Autodesk Inventor part; units mm, degrees
ref_plane "YZ Plane" through (0, 0, 0) normal (1, 0, 0) x (0, 1, 0)
ref_plane "XZ Plane" through (0, 0, 0) normal (0, 1, 0) x (-1, 0, 0)
ref_plane "XY Plane" through (0, 0, 0) normal (0, 0, 1) x (1, 0, 0)
sketch "Boceto1" plane through (0, 0, 0) normal (0, 1, 0) x (-1, 0, 0)
  line L0 (27.5, -17.5) -> (-27.5, -17.5)
  line L1 (-27.5, -17.5) -> (-27.5, 17.5)
  line L2 (-27.5, 17.5) -> (27.5, 17.5)
  line L3 (27.5, 17.5) -> (27.5, -17.5)
  line L4 (27.5, -17.5) -> (-27.5, 17.5) construction
  line L5 (-27.5, -17.5) -> (27.5, 17.5) construction
  point P0 (0, 0)
  dimension "d0" = 55
  dimension "d1" = 35
extrude "Extrusión1" add sketch "Boceto1" along normal blind 15
sketch "Boceto2" plane through (0, 15, 0) normal (0, 1, 0) x (1, 0, 0)
  line L0 (25.5, -15.5) -> (-25.5, -15.5)
  line L1 (-25.5, -15.5) -> (-25.5, 15.5)
  line L2 (-25.5, 15.5) -> (25.5, 15.5)
  line L3 (25.5, 15.5) -> (25.5, -15.5)
  line L4 (25.5, -15.5) -> (-25.5, 15.5) construction
  line L5 (-25.5, -15.5) -> (25.5, 15.5) construction
  point P0 (0, 0)
  dimension "d4" = 51
  dimension "d5" = 31
extrude "Extrusión2" cut sketch "Boceto2" against normal blind 13
sketch "Boceto3" plane through (-27.5, 0, -17.5) normal (-1, 0, 0) x (0, 0, 1)
  point P0 (17.5, 0)
sketch "Boceto4" plane through (0, 15, 0) normal (0, 1, 0) x (1, 0, 0)
  line L0 (-27.5, 17.5) -> (-27.5, -17.5)
  line L1 (-27.5, -17.5) -> (-29.5, -17.5)
  line L2 (-29.5, -17.5) -> (-29.5, 17.5)
  line L3 (-29.5, 17.5) -> (-27.5, 17.5)
  line L4 (-27.5, 17.5) -> (-27.5, -17.5)
  point P0 (0, 0)
  dimension "d8" = 2
extrude "Extrusión3" add sketch "Boceto4" against normal blind 15
sketch "Boceto5" plane through (-29.5, 15, -17.5) normal (-1, 0, 0) x (0, 0, 1)
  line L0 (35, 0) -> (0, 0)
  line L1 (0, 0) -> (9, 0)
  line L2 (9, 0) -> (9, -6.5)
  line L3 (2, -13) -> (33, -13)
  circle A0 centre (9, -6.5) radius 5.5
  point P0 (17.5, -15)
  dimension "d11" = 9
  dimension "d12" = 6.5
  dimension "d13" = 11
extrude "Extrusión4" cut sketch "Boceto5" against normal blind 2
sketch "Boceto6" plane through (-27.5, 8.5, -8.5) normal (-1, 0, 0) x (0, 0, 1)
  circle A0 centre (0, 0) radius 4
  point P0 (8.5, -8.5)
  dimension "d16" = 8
extrude "Extrusión5" cut sketch "Boceto6" against normal blind 2
sketch "Boceto7" plane through (0, 2, 0) normal (0, 1, 0) x (1, 0, 0)
  line L0 (-27.5, 3) -> (-27.5, 14)
  line L1 (-27.5, 3) -> (-27.5, 8.5)
  line L2 (-25.5, -15.5) -> (-25.5, 15.5)
  line L3 (-25.5, 8.5) -> (-25.5, 1.5)
  line L4 (-25.5, 15.5) -> (25.5, 15.5)
  line L5 (7.5, 15.5) -> (7.5, 14.5)
  line L6 (7.5, 14.5) -> (6.5, 14.5)
  line L7 (6.5, 14.5) -> (6.5, 15.5)
  line L8 (6.5, 1.5) -> (6.5, 2.5547)
  line L9 (6.5, 2.5547) -> (7.5, 2.5547)
  line L10 (7.5, 2.5547) -> (7.5, 0.5)
  line L11 (7.5, 0.5) -> (-5.5, 0.5)
  line L12 (-5.5, 0.5) -> (-5.5, 1.5)
  line L13 (-5.5, 1.5) -> (6.5, 1.5)
  point P0 (0, 0)
  dimension "d19" = 7
  dimension "d27" = 32
extrude "Extrusión6" add sketch "Boceto7" along normal blind 13 contours L8 L9 L10 L11 L12 L13
sketch "Boceto8" plane through (0, 2, 0) normal (0, 1, 0) x (1, 0, 0)
  line L0 (6.5, 1.5) -> (6.5, 2.5547)
  line L1 (-25.5, 15.5) -> (25.5, 15.5)
  line L2 (6.5, 15.5) -> (6.5, 14.5)
  line L3 (6.5, 14.5) -> (7.5, 14.5)
  line L4 (7.5, 14.5) -> (7.5, 15.5)
  point P0 (0, 0)
extrude "Extrusión7" add sketch "Boceto8" along normal blind 13
sketch "Boceto9" plane through (0, 15, 0) normal (0, 1, 0) x (1, 0, 0)
  line L0 (-29.5, -17.5) -> (27.5, -17.5)
  line L1 (27.5, -17.5) -> (27.5, -21.5)
  line L2 (27.5, -21.5) -> (-29.5, -21.5)
  line L3 (-29.5, -21.5) -> (-29.5, -17.5)
  point P0 (0, 0)
  dimension "d34" = 4
extrude "Extrusión8" add sketch "Boceto9" against normal blind 15
sketch "Boceto10" plane through (0, 15, 0) normal (0, 1, 0) x (1, 0, 0)
  line L0 (25.5, -15.5) -> (-25.5, -15.5)
  line L1 (-25.5, -15.5) -> (25.5, -15.5)
  line L2 (25.5, -15.5) -> (25.5, -19.5)
  line L3 (25.5, -19.5) -> (-25.5, -19.5)
  line L4 (-25.5, -19.5) -> (-25.5, -15.5)
  point P0 (0, 0)
  dimension "d37" = 4
extrude "Extrusión9" cut sketch "Boceto10" against normal blind 13
sketch "Boceto11" plane through (-29.5, 0, -17.5) normal (-1, 0, 0) x (0, 0, 1)
  line L0 (39, 15) -> (37, 15)
  line L1 (39, 15) -> (0, 15)
  line L2 (37, 15) -> (27, 15)
  line L3 (0, 0) -> (39, 0)
  line L4 (2, 2) -> (37, 2)
  line L5 (27, 5.5) -> (27, 8.5)
  line L6 (27, 5.5) -> (31, 5.5)
  line L7 (31, 5.5) -> (31, 2.5)
  line L8 (31, 2.5) -> (23, 2.5)
  line L9 (23, 2.5) -> (23, 5.5)
  line L10 (23, 5.5) -> (27, 5.5)
  point P0 (17.5, 0)
  dimension "d41" = 10
  dimension "d45" = 3
  dimension "d46" = 4
extrude "Extrusión10" cut sketch "Boceto11" against normal blind 4
sketch "Boceto12" plane through (-25.5, 2, -15.5) normal (1, 0, 0) x (0, 0, -1)
  line L0 (-29, 3.5) -> (-29, 0.5)
  line L1 (-29, 3.5) -> (-25, 3.5)
  line L2 (-29, 3.5) -> (-21, 3.5)
  line L3 (-25, 6.5) -> (-21, 6.5)
  line L4 (-21, 0.5) -> (-21, 3.5)
  line L5 (-21, 6.5) -> (-21, 3.5)
  line L6 (-21, 3.5) -> (-29, 3.5)
  line L7 (-29, 6.5) -> (-29, 3.2703)
  line L8 (-29, 6.5) -> (-25, 6.5)
  point P0 (-15.5, -2)
sketch "Boceto13" plane through (-25.5, 2, -15.5) normal (1, 0, 0) x (0, 0, -1)
  line L0 (-25, 3.524) -> (-34.5, 3.524)
  line L1 (-35, 13) -> (-35, 0)
  line L2 (-34.5, 3.524) -> (-34.5, 6.524)
  line L3 (-35, 13) -> (0, 13)
  line L4 (-34.5, 6.524) -> (-15.5, 6.524)
  line L5 (-15.5, 6.524) -> (-15.5, 3.524)
  line L6 (-35, 0) -> (0, 0)
  line L7 (-15.5, 3.524) -> (-25, 3.524)
  point P0 (-15.5, -2)
  dimension "d52" = 9.5
  dimension "d54" = 3
  dimension "d55" = 19
  dimension "d56" = 3
extrude "Extrusión11" cut sketch "Boceto13" against normal blind 2
sketch "Boceto14" plane through (27.5, 0, -17.5) normal (1, 0, 0) x (0, 0, -1)
  line L0 (0, 15) -> (0, 0)
  line L1 (0, 0) -> (-19.5, 0)
  line L2 (-39, 0) -> (0, 0)
  line L3 (-19.5, 0) -> (-19.5, 7.5)
  line L4 (-36.5, 8.524) -> (-17.5, 8.524)
  line L5 (-19.5, 7.5) -> (-24.5, 7.5)
  line L6 (-39, 15) -> (-39, 0)
  line L7 (-24.5, 7.5) -> (-24.5, 6.5)
  line L8 (-24.5, 6.5) -> (-14.5, 6.5)
  line L9 (-14.5, 6.5) -> (-14.5, 8.5)
  line L10 (-37, 15) -> (-2, 15)
  line L11 (-24.5, 6.5) -> (-24.5, 8.5)
  line L12 (-24.5, 8.5) -> (-14.5, 8.5)
  point P0 (-17.5, 0)
  dimension "d59" = 19.5
  dimension "d60" = 7.5
  dimension "d61" = 5
  dimension "d62" = 1
  dimension "d63" = 10
  dimension "d64" = 2
  dimension "d65" = 2
extrude "Extrusión12" cut sketch "Boceto14" against normal blind 3
sketch "Boceto15" plane through (0, 15, 0) normal (0, 1, 0) x (1, 0, 0)
  line L0 (27.5, -21.5) -> (-29.5, -21.5)
  line L1 (27.5, 17.5) -> (-29.5, 17.5)
  line L2 (-29.5, -21.5) -> (27.5, -21.5)
  line L3 (27.5, -21.5) -> (27.5, 17.5)
  line L4 (27.5, 17.5) -> (-29.5, 17.5)
  line L5 (27.5, -21.5) -> (27.5, 17.5)
  line L6 (27.5, 17.5) -> (27.5, 16.5)
  line L7 (26.5, 16.5) -> (-28.5, 16.5)
  line L8 (-28.5, -20.5) -> (26.5, -20.5)
  line L9 (26.5, -20.5) -> (26.5, 16.5)
  line L10 (-28.5, 16.5) -> (-29.5, 16.5)
  line L11 (-29.5, 17.5) -> (-29.5, -21.5)
  line L12 (27.5, 17.5) -> (-29.5, 17.5)
  line L13 (-29.5, 16.5) -> (-29.5, 17.5)
  line L14 (-28.5, -20.5) -> (-29.5, -20.5)
  line L15 (-29.5, -21.5) -> (-29.5, -20.5)
  point P0 (0, 0)
  dimension "d69" = 1
  dimension "d70" = 55
  dimension "d71" = 37
sketch "Boceto16" plane through (0, 15, 0) normal (0, 1, 0) x (1, 0, 0)
  point P0 (0, 0)
extrude "Extrusión13" cut sketch "Boceto15" against normal blind 3 contours L0 L11 L14 L8 L9 L7 L10 L1 L3
sketch "Boceto17" plane through (-29.5, 15, 20.5) normal (0, 0, 1) x (1, 0, 0)
  line L0 (0, 0) -> (56, 0)
  line L1 (56, 0) -> (56, -3)
  line L2 (0, 0) -> (56, 0)
  line L3 (56, 0) -> (56, -1.5)
  line L4 (56, -1.5) -> (0, -1.5)
  line L5 (0, -1.5) -> (0, 0)
  point P0 (29.5, -15)
extrude "Extrusión14" add sketch "Boceto17" along normal blind 1
sketch "Boceto18" plane through (26.5, 15, -16.5) normal (0, 0, -1) x (-1, 0, 0)
  line L0 (0, 0) -> (56, 0)
  line L1 (0, -1.5) -> (56, -1.5)
  line L2 (0, 0) -> (56, 0)
  line L3 (56, 0) -> (56, -1.5)
  line L4 (56, -1.5) -> (0, -1.5)
  line L5 (0, -1.5) -> (0, 0)
  point P0 (26.5, -15)
extrude "Extrusión15" add sketch "Boceto18" along normal blind 1
sketch "Boceto19" plane through (-29.5, 0, -17.5) normal (-1, 0, 0) x (0, 0, 1)
  line L0 (23, 2.5) -> (23, 5.5)
  line L1 (23, 5.5) -> (31, 5.5)
  line L2 (31, 5.5) -> (31, 8.5)
  line L3 (31, 8.5) -> (23, 8.5)
  line L4 (23, 8.5) -> (23, 5.5)
  point P0 (17.5, 0)
  dimension "d78" = 8
  dimension "d79" = 3
extrude "Extrusión16" cut sketch "Boceto19" against normal blind 6
sketch "Boceto20" plane through (-29.5, 0, -17.5) normal (-1, 0, 0) x (0, 0, 1)
  line L0 (23, 8.5) -> (23, 5.524)
  line L1 (23, 8.5) -> (22.5, 8.5)
  line L2 (24.5, 8.5) -> (14.5, 8.5)
  line L3 (22.5, 8.5) -> (22.5, 2.5)
  line L4 (22.5, 2.5) -> (31.5, 2.5)
  line L5 (23, 2.5) -> (31, 2.5)
  line L6 (31.5, 2.5) -> (31.5, 8.5)
  line L7 (31.5, 8.5) -> (22.5, 8.5)
  point P0 (17.5, 0)
  dimension "d82" = 0.5
  dimension "d83" = 6
  dimension "d84" = 9
  dimension "d85" = 6
extrude "Extrusión17" cut sketch "Boceto20" against normal blind 6
sketch "Boceto21" plane through (-25.5, 2, -15.5) normal (1, 0, 0) x (0, 0, -1)
  line L0 (-34.5, 6.524) -> (-15.5, 6.524)
  line L1 (-34.5, 6.524) -> (-34.5, 7.524)
  line L2 (-34.5, 7.524) -> (-15.5, 7.524)
  line L3 (-15.5, 7.524) -> (-15.5, 6.524)
  line L4 (-15.5, 6.524) -> (-34.5, 6.524)
  point P0 (-15.5, -2)
  dimension "d88" = 1
extrude "Extrusión18" cut sketch "Boceto21" against normal blind 2
sketch "Boceto22" plane through (26.5, 12, 20.5) normal (1, 0, 0) x (0, 0, -1)
  line L0 (0, 0) -> (37, 0)
  line L1 (37, 0) -> (37, 3)
  line L2 (-1, 3) -> (38, 3)
  line L3 (37, 3) -> (38, 3)
  line L4 (37, 0) -> (38, 0)
  line L5 (38, 3) -> (38, 0)
  line L6 (38, 0) -> (37, 0)
  line L7 (0, 1.5) -> (0, 0)
  line L8 (-1, 0) -> (-1, -12)
  line L9 (0, 0) -> (-1, 0)
  line L10 (-1, 0) -> (-1, 3)
  line L11 (0, 3) -> (0, 0)
  point P0 (20.5, -12)
extrude "Extrusión19" cut sketch "Boceto22" against normal blind 100 contours L9 L10 L2 L11 L7 | L1 L2 L5 L4
sketch "Boceto23" plane through (26.5, 15, 20.5) normal (1, 0, 0) x (0, 0, -1)
  line L0 (37, 0) -> (37, -3)
  line L1 (37, 0) -> (38, 0)
  line L2 (38, 0) -> (38.5, 0)
  line L3 (38.5, 0) -> (38.5, 1)
  line L4 (38.5, 1) -> (37, 1)
  line L5 (37, 1) -> (36, 1)
  line L6 (36, 1) -> (36, 0)
  line L7 (37, 0) -> (36, 0)
  line L8 (0, 0) -> (37, 0)
  point P0 (20.5, -15)
  dimension "d93" = 1
  dimension "d94" = 0.5
  dimension "d95" = 1
extrude "Extrusión20" add sketch "Boceto23" against normal blind 56
sketch "Boceto24" plane through (26.5, 15, 20.5) normal (1, 0, 0) x (0, 0, -1)
  line L0 (36, 0) -> (0, 0)
  line L1 (0, 0) -> (-1.5, 0)
  line L2 (-1.5, 0) -> (-1.5, 1)
  line L3 (-1.5, 1) -> (0.5, 1)
  line L4 (0.5, 1) -> (1, 1)
  line L5 (1, 0) -> (36, 0)
  line L6 (1, 1) -> (1, 0)
  line L7 (1, 0) -> (0, 0)
  point P0 (20.5, -15)
  dimension "d98" = 1.5
  dimension "d99" = 1
  dimension "d100" = 2
  dimension "d101" = 0.5
extrude "Extrusión21" add sketch "Boceto24" against normal blind 56
sketch "Boceto25" plane through (26.5, 15, 19.5) normal (1, 0, 0) x (0, 0, -1)
  line L0 (-2.5, 1) -> (0, 1)
  line L1 (-1, 0) -> (-2.5, 0)
  line L2 (-2.5, 1) -> (-2, 1)
  line L3 (-2, 1) -> (-2, 0)
  line L4 (-2, 0) -> (-2.5, 0)
  line L5 (-2.5, 0) -> (-2.5, 1)
  line L6 (37.5, 1) -> (35, 1)
  line L7 (36, 0) -> (37.5, 0)
  line L8 (37.5, 1) -> (37, 1)
  line L9 (37, 1) -> (37, 0)
  line L10 (37, 0) -> (37.5, 0)
  line L11 (37.5, 0) -> (37.5, 1)
  point P0 (19.5, -15)
  point P1 (-2, 1)
  dimension "d104" = 0.5
  dimension "d105" = 0.5
extrude "Extrusión22" cut sketch "Boceto25" against normal blind 56
sketch "Boceto26" plane through (26.5, 15, 19.5) normal (1, 0, 0) x (0, 0, -1)
  point P0 (19.5, -15)
sketch "Boceto27" plane through (26.5, 15, 19.5) normal (1, 0, 0) x (0, 0, -1)
  line L0 (35, 0) -> (0, 0)
  line L1 (0, 1) -> (0, 0)
  line L2 (35, 0) -> (0, 0)
  line L3 (0, 0) -> (0, 1)
  line L4 (0, 1) -> (35, 1)
  line L5 (35, 1) -> (35, 0)
  point P0 (19.5, -15)
extrude "Extrusión23" add sketch "Boceto27" against normal blind 1
properties part number "CajaArduinoNano"
Geometry check sheet. Reference: the model listing, model coordinates, mm. A direction names the side the tool comes from. Coordinates: 2 decimals unless noted, no trailing zeros. Order: outer loops, then holes, each group sorted by start corner. A loop starts at its lowest first (then second) coordinate and runs counter-clockwise, first axis right, second up. Notation, with made-up numbers: (66.5, 28.25) - (95.5, 28.25) arc R25 ccw to (95.5, 43.25) - close; hole circle Ø4 at (20.25, -17.5). An arc over 180 degrees is marked (long way). Answer in a Markdown table with one row per item. Add a question column.
1) Gauge pin test, flat ends, axial feed: P1, Ø1.5, axis at x = -10, z = -1.5, coming from the +Y side; P2, Ø3, axis at x = -27, z = 9.5, coming from the +Y side; P3, Ø5, axis at y = 8.5, z = -8.5, coming from the -X side. Record the tip position at first contact, or that the pin passes through.
2) Cross-section at C-C, the plane z = 15.5. Record the cut outline in (x, y).
3) Cross-section at B-B, the plane x = 16. Record the cut outline in (y, z), then the cut area to 3 significant figures.
4) Material ranges on line 1 along X through (y, z) = (11.75, -15); line 2 along X through (y, z) = (12.5, 3); line 3 along X through (y, z) = (8, -13), recorded low to high. Write a range as [from, to].
5) Set-up check for faces 1 (the flat face through (25.5, 9, 2)), 2 (the flat face through (1, 15, -1)), 3 (the flat face through (-27.5, 4, -8)): record each of +Z, -Z, +X, -X, +Y, -Y from which the full face is reachable in a straight line by a thin tool's end or side.
6) Release check for a two-part mould opening along Z. For faces 4 (the flat face through (-26, 9.524, 10)), 5 (the flat face through (-1, 0, 2)), 6 (the flat face through (-1, 14, 20.5)) record: +Z half, -Z half, draft (parallel to the pull), parting line (faces both ways), or undercut.
7) Cross-section at D-D, the plane z = -8.5. Record the cut outline in (x, y), then the cut area to 3 significant figures.
8) Cross-section at A-A, the plane z = 2. Record the cut outline in (x, y).
Check result:
| question | item | result |
|---|---|---|
| 1 | P1 | stops at y = 2 |
| 1 | P2 | stops at y = 15 |
| 1 | P3 | stops at x = 25.5 |
| 2 | outline | (-29.5, 0) - (27.5, 0) - (27.5, 12) - (26.5, 12) - (26.5, 16) - (25.5, 16) - (25.5, 2) - (-25.5, 2) - (-25.5, 5.52) - (-27.5, 5.52) - (-27.5, 9.52) - (-25.5, 9.52) - (-25.5, 15) - (-29.5, 15) - close |
| 3 | outline | (0, -17.5) - (12, -17.5) - (12, -16.5) - (15, -16.5) - (15, -17.5) - (16, -17.5) - (16, -15.5) - (2, -15.5) - (2, 19.5) - (16, 19.5) - (16, 21.5) - (15, 21.5) - (15, 20.5) - (12, 20.5) - (12, 21.5) - (0, 21.5) - close |
| 3 | area | 128 mm² |
| 4 | line 1 | x = [-29.5, -25.5], [6.5, 7.5], [25.5, 27.5] |
| 4 | line 2 | x = [-29.5, -25.5], [25.5, 26.5] |
| 4 | line 3 | x = [-27.5, -25.5], [25.5, 27.5] |
| 5 | face 1 | +Y |
| 5 | face 2 | -X, +Y |
| 5 | face 3 | -X |
| 6 | face 4 | undercut |
| 6 | face 5 | draft |
| 6 | face 6 | +Z half |
| 7 | outline | (-29.5, 0) - (27.5, 0) - (27.5, 12) - (26.5, 12) - (26.5, 16) - (25.5, 16) - (25.5, 2) - (-25.5, 2) - (-25.5, 4.5) - (-27.5, 4.5) - (-27.5, 3) - (-29.5, 3) - close; (-29.5, 14) - (-27.5, 14) - (-27.5, 12.5) - (-25.5, 12.5) - (-25.5, 15) - (-29.5, 15) - close |
| 7 | area | 152 mm² |
| 8 | outline | (-29.5, 0) - (27.5, 0) - (27.5, 6.5) - (25.5, 6.5) - (25.5, 2) - (-25.5, 2) - (-25.5, 5.52) - (-27.5, 5.52) - (-27.5, 9.52) - (-25.5, 9.52) - (-25.5, 15) - (-29.5, 15) - close; (25.5, 8.5) - (27.5, 8.5) - (27.5, 12) - (26.5, 12) - (26.5, 16) - (25.5, 16) - close |
